The model under review builds one solid part; all positions refer to its coordinate system, in mm. A direction names the side the tool comes from. Coordinates: 2 decimals unless noted, no trailing zeros. Loops run counter-clockwise (first coordinate to the right, second up) from the corner with the lowest first, then second, coordinate; pieces in that order, holes last. Notation, with made-up numbers: (78.5, -25) - (88.5, -25) arc R18 cw to (88.5, -15) - close; hole circle Ø7 at (67, 79). An arc over 180 degrees is marked (long way). Answer in a Markdown table with one row per item. Add a question column.
(1) For line 1 along X through (y, z) = (-46.1, 10); line 2 along X through (y, z) = (45, 4.5); line 3 along Z through (x, y) = (-8, -35), list the stretches that pass through material, from the lowest coordinate up.
(2) Machinability: for faces 5 (the flat face through (4, -45.471, 11)), 6 (the flat face through (4, 3, 0)), 7 (the flat face through (4, -46.371, 10)), which of the approach directions +Z, -Z, +X, -X, +Y, -Y give a long, thin tool a straight path to every point of the face, cutting with its end or side? Answer none if there is none.
(3) We need section C-C on y = -23. Write out the cut boundary in (x, z), plus the area to 3 significant figures.
(4) We need section A-A on y = 35.5. Write out the cut boundary in (x, z).
(5) For P1, Ø1, axis at y = -45.5, z = 11.5, coming from the +X side; P2, Ø5, axis at x = -9.5, y = 53, coming from the +Z side; P3, Ø2, axis at x = -11, z = 3, coming from the +Y side, all flat-tipped, find the tip position at first contact; note any pin that passes through.
(6) Mouldability with a two-part tool opening along Z and no side actions: class faces 1 (the cylindrical face through (-6.66, -45.93, 11.28)), 2 (the cylindrical face through (14.716, -45.928, 10.807)), 3 (the flat face through (4, 3, -0.9)), 4 (the flat face through (-18.337, 16, 6)) as +Z half, -Z half, draft (parallel to the pull), parting line (faces both ways), or undercut.
(7) We need section B-B on z = 4. Write out the cut boundary in (x, y), plus the area to 4 significant figures.
(8) We need section D-D on x = 6.5. Write out the cut boundary in (y, z).
from build123d import *

# Parameters (mm, degrees)
SKETCH1_W                    = 45
SKETCH1_H                    = 120
BASE_FLANGE2_DEPTH           = 0.9
EDGE_FLANGE2_DEPTH           = 45
SKETCH17_W                   = 15
SKETCH17_H                   = 60
CUT_EXTRUDE1_DEPTH           = 10
EDGE_FLANGE4_STRIP_W         = 5.6
EDGE_FLANGE4_STRIP_H         = 0.9
EDGE_FLANGE4_STRIP_CUT_DEPTH = 120
EDGE_FLANGE4_DEPTH           = 120
EDGE_FLANGE5_STRIP_W         = 5.6
EDGE_FLANGE5_STRIP_H         = 0.9
EDGE_FLANGE5_STRIP_CUT_DEPTH = 120
EDGE_FLANGE5_DEPTH           = 120
F_19_0_166_DIAMETER_SLOT2_D  = 4.2164
F_19_0_166_DIAMETER_SLOT1_D  = 4.2164


# Sheet-metal steps are written as plain solids
with BuildPart() as part:
    # Sketch1 → Base-Flange2 (new body)
    with BuildSketch(Plane.XY):
        with Locations((4.162995595, 15.528634361)):
            Rectangle(SKETCH1_W, SKETCH1_H)
    extrude(amount=-BASE_FLANGE2_DEPTH)

    # Edge-Flange2 section (across the edge) → Edge-Flange2 (add)
    with BuildSketch(Plane(origin=(-18.337004405, -45.471365639, 0), x_dir=(0, 1, 0), z_dir=(1, 0, 0))):
        with BuildLine():
            Line((-0.9, 1), (-0.9, 20))
            Line((-0.9, 20), (0, 20))
            Line((0, 20), (0, 1))
            ThreePointArc((0, 1), (0.292893219, 0.292893219), (1, 0))
            Line((1, 0), (1, -0.9))
            ThreePointArc((1, -0.9), (-0.343502884, -0.343502884), (-0.9, 1))
        make_face()
    extrude(amount=EDGE_FLANGE2_DEPTH)

    # Sketch17 → Cut-Extrude1 (cut)
    with BuildSketch(Plane.XY):
        with Locations((4.162995595, 45.528634361)):
            Rectangle(SKETCH17_W, SKETCH17_H)
    extrude(amount=-CUT_EXTRUDE1_DEPTH, mode=Mode.SUBTRACT)

    # Edge-Flange4 strip (across the edge) → Edge-Flange4 strip cut (cut)
    with BuildSketch(Plane(origin=(-18.337004405, 75.528634361, 0), x_dir=(1, 0, 0), z_dir=(0, -1, 0))):
        with Locations((-1.8, -0.45)):
            Rectangle(EDGE_FLANGE4_STRIP_W, EDGE_FLANGE4_STRIP_H)
    extrude(amount=EDGE_FLANGE4_STRIP_CUT_DEPTH, mode=Mode.SUBTRACT)

    # Edge-Flange4 section (across the edge) → Edge-Flange4 (add)
    with BuildSketch(Plane(origin=(-18.337004405, 75.528634361, 0), x_dir=(1, 0, 0), z_dir=(0, -1, 0))):
        with BuildLine():
            Line((-0.9, 1), (-0.9, 10))
            Line((-0.9, 10), (0, 10))
            Line((0, 10), (0, 1))
            ThreePointArc((0, 1), (0.292893219, 0.292893219), (1, 0))
            Line((1, 0), (1, -0.9))
            ThreePointArc((1, -0.9), (-0.343502884, -0.343502884), (-0.9, 1))
        make_face()
    extrude(amount=EDGE_FLANGE4_DEPTH)

    # Edge-Flange5 strip (across the edge) → Edge-Flange5 strip cut (cut)
    with BuildSketch(Plane(origin=(26.662995595, -44.471365639, 0), x_dir=(-1, 0, 0), z_dir=(0, 1, 0))):
        with Locations((-1.8, -0.45)):
            Rectangle(EDGE_FLANGE5_STRIP_W, EDGE_FLANGE5_STRIP_H)
    extrude(amount=EDGE_FLANGE5_STRIP_CUT_DEPTH, mode=Mode.SUBTRACT)

    # Edge-Flange5 section (across the edge) → Edge-Flange5 (add)
    with BuildSketch(Plane(origin=(26.662995595, -44.471365639, 0), x_dir=(-1, 0, 0), z_dir=(0, 1, 0))):
        with BuildLine():
            Line((-0.9, 1), (-0.9, 10))
            Line((-0.9, 10), (0, 10))
            Line((0, 10), (0, 1))
            ThreePointArc((0, 1), (0.292893219, 0.292893219), (1, 0))
            Line((1, 0), (1, -0.9))
            ThreePointArc((1, -0.9), (-0.343502884, -0.343502884), (-0.9, 1))
        make_face()
    extrude(amount=EDGE_FLANGE5_DEPTH)

    # #19 (0.166) Diameter Slot2 (through all)
    with Locations(Plane(origin=(0, -45.471365639, 0), x_dir=(1, 0, 0), z_dir=(0, 1, 0))):
        with Locations((16.662995595, -10), (-8.337004405, -10)):
            Hole(F_19_0_166_DIAMETER_SLOT2_D / 2)

    # #19 (0.166) Diameter Slot1 (through all)
    with Locations(Plane.XY):
        with Locations((3.27299702, -3.085765259)):
            Hole(F_19_0_166_DIAMETER_SLOT1_D / 2)


solid = part.part
Outcome:
| question | item | result |
|---|---|---|
| 1 | line 1 | -18.34 to -10.45, -6.23 to 14.55, 18.77 to 26.66 |
| 1 | line 2 | -19.24 to -18.34, 26.66 to 27.56 |
| 1 | line 3 | -0.9 to 0 |
| 2 | face 5 | +Z, +X, -X, +Y |
| 2 | face 6 | +Z, +Y |
| 2 | face 7 | +Z, -Z, +X, -X, -Y |
| 3 | outline | (-19.24, 1) arc R1.9 ccw to (-17.34, -0.9) - (25.66, -0.9) arc R1.9 ccw to (27.56, 1) - (27.56, 10) - (26.66, 10) - (26.66, 1) arc R1 cw to (25.66, 0) - (-17.34, 0) arc R1 cw to (-18.34, 1) - (-18.34, 10) - (-19.24, 10) - close |
| 3 | area | 59.0 mm² |
| 4 | outline | (-19.24, 1) arc R1.9 ccw to (-17.34, -0.9) - (-3.34, -0.9) - (-3.34, 0) - (-17.34, 0) arc R1 cw to (-18.34, 1) - (-18.34, 10) - (-19.24, 10) - close; (11.66, -0.9) - (25.66, -0.9) arc R1.9 ccw to (27.56, 1) - (27.56, 10) - (26.66, 10) - (26.66, 1) arc R1 cw to (25.66, 0) - (11.66, 0) - close |
| 5 | P1 | x = 26.66 |
| 5 | P2 | z = 0 |
| 5 | P3 | y = -45.47 |
| 6 | face 1 | undercut |
| 6 | face 2 | undercut |
| 6 | face 3 | -Z half |
| 6 | face 4 | draft |
| 7 | outline | (-19.24, -44.47) - (-18.34, -44.47) - (-18.34, 75.53) - (-19.24, 75.53) - close; (-18.34, -46.37) - (26.66, -46.37) - (26.66, -45.47) - (-18.34, -45.47) - close; (26.66, -44.47) - (27.56, -44.47) - (27.56, 75.53) - (26.66, 75.53) - close |
| 7 | area | 256.5 mm² |
| 8 | outline | (-46.37, 1) arc R1.9 ccw to (-44.47, -0.9) - (15.53, -0.9) - (15.53, 0) - (-44.47, 0) arc R1 cw to (-45.47, 1) - (-45.47, 20) - (-46.37, 20) - close |
